from build123d import *

# Parameters (mm, degrees)
SKETCH_2_W          = 80
SKETCH_2_H          = 24
SKETCH_2_W_2        = 78
SKETCH_2_H_2        = 22
EXTRUDE_3130_DEPTH  = 20.5
SKETCH_2_3_W        = 10
SKETCH_2_3_H        = 22
SKETCH_2_3_R        = 1.5
SKETCH_2_3_W_2      = 46
SKETCH_2_3_R_2      = 2
SKETCH_2_3_W_3      = 4
SKETCH_2_3_H_2      = 8
SKETCH_2_3_W_4      = 12.2
SKETCH_2_3_H_3      = 27
EXTRUDE_3218_DEPTH  = 1
CUT_EXTRUDE_START   = -18.7
SKETCH_3_R          = 1.5
CUT_EXTRUDE_1_DEPTH = 14.6
CUT_EXTRUDE_START_2 = -48.8
SKETCH_3_2_R        = 1.5
SKETCH_3_2_W        = 8
SKETCH_3_2_H        = 8
CUT_EXTRUDE_2_DEPTH = 1.2
SKETCH_2_5_W        = 1
SKETCH_2_5_H        = 22
EXTRUDE_4_DEPTH     = 8


with BuildPart() as part:
    # Эскиз2 → Extrude 3130 (new body)
    # profile 1 of 8: a face of its own
    with BuildSketch(Plane(origin=(0, 0, 0), x_dir=(1, 0, 0), z_dir=(0, 1, 0))):
        Rectangle(SKETCH_2_W, SKETCH_2_H)
        Rectangle(SKETCH_2_W_2, SKETCH_2_H_2, mode=Mode.SUBTRACT)
    # profile 2 of 8: a face of its own
    with BuildSketch(Plane(origin=(0, 0, 0), x_dir=(1, 0, 0), z_dir=(0, 1, 0))):
        with BuildLine():
            Line((-33.3, -39), (-32.1, -39))
            Line((-32.1, -39), (-32.1, -12))
            Line((-32.1, -12), (-33.3, -12))
            Line((-33.3, -12), (-33.3, -22.903910844))
            ThreePointArc((-33.3, -22.903910844), (-39.756802154, -15.868113034), (-48.8, -12.8))
            Line((-48.8, -12.8), (-48.8, 12.8))
            ThreePointArc((-48.8, 12.8), (-39.756802154, 15.868113034), (-33.3, 22.903910844))
            Line((-33.3, 22.903910844), (-33.3, 12))
            Line((-33.3, 12), (-32.1, 12))
            Line((-32.1, 12), (-32.1, 39))
            Line((-32.1, 39), (-33.3, 39))
            Line((-33.3, 39), (-33.3, 26))
            ThreePointArc((-33.3, 26), (-39.767640231, 17.380382655), (-50, 14))
            Line((-50, 14), (-50, -14))
            ThreePointArc((-50, -14), (-39.767640231, -17.380382655), (-33.3, -26))
            Line((-33.3, -26), (-33.3, -39))
        make_face()
    # profile 3 of 8: a face of its own
    with BuildSketch(Plane(origin=(0, 0, 0), x_dir=(1, 0, 0), z_dir=(0, 1, 0))):
        Polygon((-18.7, 34), (-18.7, 34.8), (-18.7, 39), (-19.9, 39), (-19.9, 12), (-18.7, 12), align=None)
    # profile 4 of 8: a face of its own
    with BuildSketch(Plane(origin=(0, 0, 0), x_dir=(1, 0, 0), z_dir=(0, 1, 0))):
        Polygon((-18.7, -39), (-18.7, -34.8), (-18.7, -34), (-18.7, -12), (-19.9, -12), (-19.9, -39), align=None)
    # profile 5 of 8: a face of its own
    with BuildSketch(Plane(origin=(0, 0, 0), x_dir=(1, 0, 0), z_dir=(0, 1, 0))):
        Polygon((28.1, 34), (28.1, 34.8), (-18.7, 34.8), (-18.7, 34), (-11.7, 34), (-10.7, 34), (27.3, 34), (27.3, 12), (28.1, 12), align=None)
    # profile 6 of 8: a face of its own
    with BuildSketch(Plane(origin=(0, 0, 0), x_dir=(1, 0, 0), z_dir=(0, 1, 0))):
        with BuildLine():
            Line((39, 12), (40, 12))
            add(Edge.make_bspline(
                [(28.1, 34.8), (40.01829159, 27.087388808), (40, 12)],
                knots=[0, 0, 0, 1, 1, 1], degree=2))
            Line((28.1, 34.8), (28.1, 34))
            add(Edge.make_bspline(
                [(28.1, 34), (35.667325964, 28.510032971), (38.830570785, 20.077982561), (39, 12)],
                knots=[0, 0, 0, 0, 1, 1, 1, 1], degree=3))
        make_face()
    # profile 7 of 8: a face of its own
    with BuildSketch(Plane(origin=(0, 0, 0), x_dir=(1, 0, 0), z_dir=(0, 1, 0))):
        Polygon((-18.7, -34.8), (28.1, -34.8), (28.1, -34), (28.1, -12), (27.3, -12), (27.3, -34), (-18.7, -34), align=None)
    # profile 8 of 8: a face of its own
    with BuildSketch(Plane(origin=(0, 0, 0), x_dir=(1, 0, 0), z_dir=(0, 1, 0))):
        with BuildLine():
            add(Edge.make_bspline(
                [(28.1, -34.8), (40.01829159, -27.087388808), (40, -12)],
                knots=[0, 0, 0, 1, 1, 1], degree=2))
            Line((40, -12), (39, -12))
            add(Edge.make_bspline(
                [(28.1, -34), (35.667325964, -28.510032971), (38.830570785, -20.077982561), (39, -12)],
                knots=[0, 0, 0, 0, 1, 1, 1, 1], degree=3))
            Line((28.1, -34), (28.1, -34.8))
        make_face()
    extrude(amount=EXTRUDE_3130_DEPTH)

    # Эскиз2<3> → Extrude 3218 (add)
    # profile 1 of 6: a face of its own
    with BuildSketch(Plane(origin=(0, 0, 0), x_dir=(1, 0, 0), z_dir=(0, 1, 0))):
        Rectangle(SKETCH_2_3_W, SKETCH_2_3_H)
        with Locations(Location((0, 0, 0), (0, 0, 270))):
            Circle(SKETCH_2_3_R, mode=Mode.SUBTRACT)
    # profile 2 of 6: a face of its own
    with BuildSketch(Plane(origin=(0, 0, 0), x_dir=(1, 0, 0), z_dir=(0, 1, 0))):
        with Locations((4.3, -23)):
            Rectangle(SKETCH_2_3_W_2, SKETCH_2_3_H)
        with Locations(Location((24.1, -23, 0), (0, 0, 270))):
            Circle(SKETCH_2_3_R_2, mode=Mode.SUBTRACT)
    # profile 3 of 6: a face of its own
    with BuildSketch(Plane(origin=(0, 0, 0), x_dir=(1, 0, 0), z_dir=(0, 1, 0))):
        with Locations((4.3, 23)):
            Rectangle(SKETCH_2_3_W_2, SKETCH_2_3_H)
        with Locations(Location((24.1, 23, 0), (0, 0, 270))):
            Circle(SKETCH_2_3_R_2, mode=Mode.SUBTRACT)
        with Locations(Location((-15.7, 31, 0), (0, 0, 270))):
            Circle(SKETCH_2_3_R, mode=Mode.SUBTRACT)
        with Locations(Location((-15.7, 16, 0), (0, 0, 270))):
            Circle(SKETCH_2_3_R, mode=Mode.SUBTRACT)
        with Locations((-15.7, 23.5)):
            Rectangle(SKETCH_2_3_W_3, SKETCH_2_3_H_2, mode=Mode.SUBTRACT)
    # profile 4 of 6: a face of its own
    with BuildSketch(Plane(origin=(0, 0, 0), x_dir=(1, 0, 0), z_dir=(0, 1, 0))):
        with Locations((-26, -25.5)):
            Rectangle(SKETCH_2_3_W_4, SKETCH_2_3_H_3)
    # profile 5 of 6: a face of its own
    with BuildSketch(Plane(origin=(0, 0, 0), x_dir=(1, 0, 0), z_dir=(0, 1, 0))):
        with Locations((-26, 25.5)):
            Rectangle(SKETCH_2_3_W_4, SKETCH_2_3_H_3)
    # profile 6 of 6: a face of its own
    with BuildSketch(Plane(origin=(0, 0, 0), x_dir=(1, 0, 0), z_dir=(0, 1, 0))):
        with BuildLine():
            Line((-33.3, -22.903910844), (-33.3, -12))
            Line((-33.3, -12), (-40, -12))
            Line((-40, -12), (-40, 12))
            Line((-40, 12), (-33.3, 12))
            Line((-33.3, 12), (-33.3, 22.903910844))
            ThreePointArc((-33.3, 22.903910844), (-39.756802154, 15.868113034), (-48.8, 12.8))
            Line((-48.8, 12.8), (-48.8, -12.8))
            ThreePointArc((-48.8, -12.8), (-39.756802154, -15.868113034), (-33.3, -22.903910844))
        make_face()
    extrude(amount=EXTRUDE_3218_DEPTH)

    # Эскиз3 → Вырез-Вытянуть1 (cut)
    with BuildSketch(Plane(origin=(0, 0, 0), x_dir=(0, 0, -1), z_dir=(1, 0, 0)).offset(CUT_EXTRUDE_START)):
        with Locations((-30, 15)):
            Circle(SKETCH_3_R)
        with Locations((30, 15)):
            Circle(SKETCH_3_R)
    extrude(amount=-CUT_EXTRUDE_1_DEPTH, mode=Mode.SUBTRACT)

    # Эскиз3<2> → Вырез-Вытянуть2 (cut)
    with BuildSketch(Plane(origin=(0, 0, 0), x_dir=(0, 0, -1), z_dir=(1, 0, 0)).offset(CUT_EXTRUDE_START_2)):
        with Locations((30, 15)):
            Circle(SKETCH_3_2_R)
        with Locations((-30, 15)):
            Circle(SKETCH_3_2_R)
        with Locations((-10, 11)):
            Circle(SKETCH_3_2_R)
        with Locations((10, 11)):
            Circle(SKETCH_3_2_R)
        with Locations((0, 11)):
            Rectangle(SKETCH_3_2_W, SKETCH_3_2_H)
    extrude(amount=-CUT_EXTRUDE_2_DEPTH, mode=Mode.SUBTRACT)

    # Эскиз2<5> → Бобышка-Вытянуть4 (add)
    with BuildSketch(Plane(origin=(0, 0, 0), x_dir=(1, 0, 0), z_dir=(0, 1, 0))):
        with Locations((-11.2, 23)):
            Rectangle(SKETCH_2_5_W, SKETCH_2_5_H)
    extrude(amount=EXTRUDE_4_DEPTH)


solid = part.part
Design review of the part built by this model. Coordinates are the model's own, in mm. A direction names the side the tool comes from. Coordinates: 2 decimals unless noted, no trailing zeros. Loops run counter-clockwise (first coordinate to the right, second up) from the corner with the lowest first, then second, coordinate; pieces in that order, holes last. Notation, with made-up numbers: (84, 71.25) -> (100, 71.25) arc R20 ccw to (100, 82.25) -> close; hole circle Ø1 at (17.25, 46.5). An arc over 180 degrees is marked (long way). Use a Markdown table: item, result. Add a question column.
Item 1: We need section D-D, the plane x = -35.5. Write out the cut boundary in (y, z).
Item 2: The part is to be moulded in two halves that separate along Z. For faces 6 (the flat face through (-33.3, 11, 17)), 7 (the flat face through (-18.7, 10, 37)), 8 (the flat face through (-26, 11, 12)), 9 (the flat face through (-19, 9, -39)), say which applies: +Z half, -Z half, draft (parallel to the pull), parting line (faces both ways), or undercut.
Item 3: We need section C-C, the plane y = 17.75. Count the separate pieces of the cut face and the enclosed holes in it, and give its area (3 significant figures).
Item 4: Clearance check with flat-ended pins moving along their axes: P1, Ø5, axis at y = 15, z = -30, coming from the -X side; P2, Ø1.1, axis at x = -16, y = 0.5, coming from the +Z side; P3, Ø1.5, axis at x = -22.5, y = 15.5, coming from the +Z side. State where each tip first meets the part, or that it passes through.
Item 5: Machinability: for faces 1 (the flat face through (-33.3, 10, -33)), 2 (the flat face through (-32.1, 11, 26)), 3 (the flat face through (-40, 11, 0)), 4 (the flat face through (-39, 10, 0)), 5 (the cylindrical face through (-19.29, 15.07, 31.5)), which of the approach directions +Z, -Z, +X, -X, +Y, -Y give a long, thin tool a straight path to every point of the face, cutting with its end or side? Answer none if there is none.
Item 6: Wall thickness on L1, parallel to Z at x = 13.5, y = 19.5; L2, parallel to X at y = 5.25, z = -0.5; L3, parallel to X at y = 2, z = -25: over which ranges is each line inside the solid? List them lowest first. Write a range as from..to.
Item 7: We need section A-A, the plane x = 0. Write out the cut boundary in (y, z).
Item 8: We need section B-B, the plane z = -3. Write out the cut boundary in (x, y), and give its area (3 significant figures).
Numbers:
| question | item | result |
|---|---|---|
| 1 | outline | (0, -21.71) -> (20.5, -21.71) -> (20.5, -19.65) -> (1, -19.65) -> (1, -12) -> (20.5, -12) -> (20.5, -11) -> (0, -11) -> close; (0, 11) -> (20.5, 11) -> (20.5, 12) -> (1, 12) -> (1, 19.65) -> (20.5, 19.65) -> (20.5, 21.71) -> (0, 21.71) -> close |
| 2 | face 6 | undercut |
| 2 | face 7 | draft |
| 2 | face 8 | +Z half |
| 2 | face 9 | -Z half |
| 3 | separate pieces | 1 |
| 3 | enclosed holes | 6 |
| 3 | area | 582 mm^2 |
| 4 | P1 | stops at x = -33.3 |
| 4 | P2 | stops at z = 34.8 |
| 4 | P3 | stops at z = 12 |
| 5 | face 1 | -Z, -X, +Y, -Y |
| 5 | face 2 | +Z, +Y |
| 5 | face 3 | +Y |
| 5 | face 4 | +Y, -Y |
| 5 | face 5 | -X |
| 6 | L1 | z = -34.8..-34, -12..-11, 11..12, 34..34.8 |
| 6 | L2 | x = -50..-48.8, -40..-39, 39..40 |
| 6 | L3 | x = -33.69..-32.1, -19.9..-18.7, -11.7..-10.7, 27.3..28.1, 35.82..37.16 |
| 7 | outline | (0, -34.8) -> (20.5, -34.8) -> (20.5, -34) -> (1, -34) -> (1, -12) -> (20.5, -12) -> (20.5, -11) -> (1, -11) -> (1, -1.5) -> (0, -1.5) -> close; (0, 1.5) -> (1, 1.5) -> (1, 11) -> (20.5, 11) -> (20.5, 12) -> (1, 12) -> (1, 34) -> (20.5, 34) -> (20.5, 34.8) -> (0, 34.8) -> close |
| 8 | outline | (-50, 0) -> (-39, 0) -> (-39, 20.5) -> (-40, 20.5) -> (-40, 1) -> (-48.8, 1) -> (-48.8, 7) -> (-50, 7) -> close; (-50, 15) -> (-48.8, 15) -> (-48.8, 20.5) -> (-50, 20.5) -> close; (-5, 0) -> (5, 0) -> (5, 1) -> (-5, 1) -> close; (39, 0) -> (40, 0) -> (40, 20.5) -> (39, 20.5) -> close |
| 8 | area | 74.8 mm^2 |
